```python
from build123d import *

# Parameters (mm, degrees)
SKETCH2_R           = 37.5
BOSS_EXTRUDE1_DEPTH = 8
CUT_EXTRUDE1_DEPTH  = 4
CIRPATTERN1_COUNT   = 3
CUT_EXTRUDE2_DEPTH  = 17
CIRPATTERN2_COUNT   = 3
SKETCH6_R           = 15
BOSS_EXTRUDE2_DEPTH = 10


with BuildPart() as part:
    # Sketch2 → Boss-Extrude1 (new body)
    with BuildSketch(Plane.XY):
        Circle(SKETCH2_R)
    extrude(amount=BOSS_EXTRUDE1_DEPTH)

    # Sketch3 → Cut-Extrude1 (cut)
    with BuildSketch(Plane.XY.offset(8)):
        Polygon((0, 23.42), (3.100370946, 25.21), (3.100370946, 28.79), (0, 30.58), (-3.100370946, 28.79), (-3.100370946, 25.21), align=None)
    cut_extrude1 = extrude(amount=-CUT_EXTRUDE1_DEPTH, mode=Mode.SUBTRACT)

    # CirPattern1: Cut-Extrude1 ×3 about axis
    cirpattern1_axis = Axis((0, 0, 0), (0, 0, 1))
    for i in range(1, CIRPATTERN1_COUNT):
        add(cut_extrude1.rotate(cirpattern1_axis, i * 360 / CIRPATTERN1_COUNT), mode=Mode.SUBTRACT)

    # Sketch5 → Cut-Extrude2 (cut)
    with BuildSketch(Plane.XY.offset(4)):
        with BuildLine():
            ThreePointArc((1.515544457, 27.875), (-0.875, 28.515544457), (-1.515544457, 26.125))
            Line((-1.515544457, 26.125), (1.515544457, 27.875))
        make_face()
        with BuildLine():
            Line((1.515544457, 27.875), (-1.515544457, 26.125))
            ThreePointArc((-1.515544457, 26.125), (0.452933329, 25.309629804), (1.75, 27))
            ThreePointArc((1.75, 27), (1.690370196, 27.452933329), (1.515544457, 27.875))
        make_face()
    cut_extrude2 = extrude(amount=-CUT_EXTRUDE2_DEPTH, mode=Mode.SUBTRACT)

    # CirPattern2: Cut-Extrude2 ×3 about axis
    cirpattern2_axis = Axis((0, 0, 0), (0, 0, 1))
    for i in range(1, CIRPATTERN2_COUNT):
        add(cut_extrude2.rotate(cirpattern2_axis, i * 360 / CIRPATTERN2_COUNT), mode=Mode.SUBTRACT)

    # Sketch6 → Boss-Extrude2 (add)
    with BuildSketch(Plane.XY.offset(8)):
        Circle(SKETCH6_R)
    extrude(amount=BOSS_EXTRUDE2_DEPTH)


solid = part.part
```
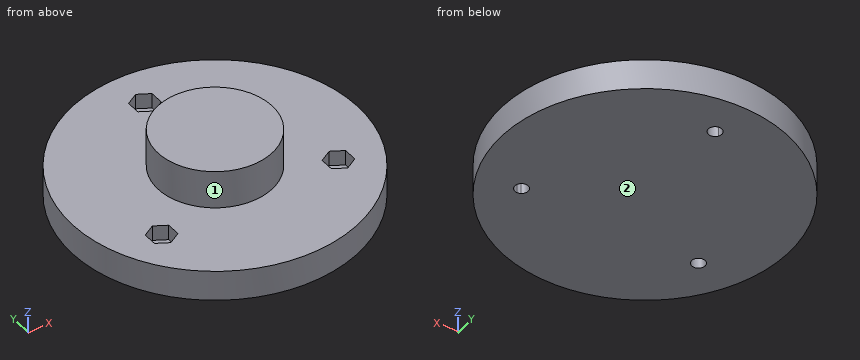
The model under review builds one solid part; all positions refer to its coordinate system, in mm. Face numbers are marked on the shaded views. A direction names the side the tool comes from. Coordinates: 2 decimals unless noted, no trailing zeros. Order: outer loops, then holes, each group sorted by start corner. A loop starts at its lowest first (then second) coordinate and runs counter-clockwise, first axis right, second up. Notation, with made-up numbers: M 36.25,57.5 L 95.25,57.5 A9 ccw 95.25,64.5 Z; hole C 27.25,29.5 d10. An arc over 180 degrees is marked long. One line per question, with ' | ' between items.
(1) Add section C-C, the plane x = -4. Write out the cut boundary in (y, z), then the cut area to 3 significant figures.
Geometry results:
outline: M -37.29,0 L 37.29,0 L 37.29,8 L 14.46,8 L 14.46,18 L -14.46,18 L -14.46,8 L -37.29,8 Z | area: 886 mm²
(2) Insertion check: pin 1 (3 mm diameter, centred on x = 23.5, y = -12, fed in from +Z); pin 2 (7 mm diameter, centred on x = -24, y = -14, fed in from +Z); pin 3 (1.5 mm diameter, centred on y = -10, z = 10, fed in from +X); pin 4 (5 mm diameter, centred on x = 13, y = -15.5, fed in from -Z). Each pin has a flat end and moves straight along its axis. Give the tip position at first contact, or say it passes through.
Geometry results:
pin 1: stops at z = 4 | pin 2: stops at z = 8 | pin 3: stops at x = 11.81 | pin 4: stops at z = 0
(3) Add section B-B, the plane y = 0. Write out the cut boundary in (x, z), then the cut area to 3 significant figures.
Geometry results:
outline: M -37.5,0 L 37.5,0 L 37.5,8 L 15,8 L 15,18 L -15,18 L -15,8 L -37.5,8 Z | area: 900 mm²
(4) Add section A-A, the plane z = 3. Write out the cut boundary in (x, y) (3 decimals).
Geometry results:
outline: C 0,0 d75; hole C -23.383,-13.5 d3.5; hole C 0,27 d3.5; hole C 23.383,-13.5 d3.5
(5) Machinability: for the marked faces 1 and 2, which of the approach directions +Z, -Z, +X, -X, +Y, -Y give a long, thin tool a straight path to every point of the face, cutting with its end or side? Answer none if there is none.
Geometry results:
face 1: +Z | face 2: -Z, +X, -X, +Y, -Y
(6) For probe 1 along X at (y, z) = (-13.5, 2.5); probe 2 along Z at (x, y) = (11.5, 31); probe 3 along Y at (x, z) = (22, 3), list the stretches that pass through material, from the lowest coordinate up. Write a range as from..to.
Geometry results:
probe 1: x = -34.99..-25.13, -21.63..21.63, 25.13..34.99 | probe 2: z = 0..8 | probe 3: y = -30.37..-14.57, -12.43..30.37
(7) Add section D-D, the plane y = -13.5. Write out the cut boundary in (x, z).
Geometry results:
outline: M -34.99,0 L -25.13,0 L -25.13,4 L -26.48,4 L -26.48,8 L -34.99,8 Z; M -21.63,0 L 21.63,0 L 21.63,4 L 20.28,4 L 20.28,8 L 6.54,8 L 6.54,18 L -6.54,18 L -6.54,8 L -20.28,8 L -20.28,4 L -21.63,4 Z; M 25.13,0 L 34.99,0 L 34.99,8 L 26.48,8 L 26.48,4 L 25.13,4 Z
